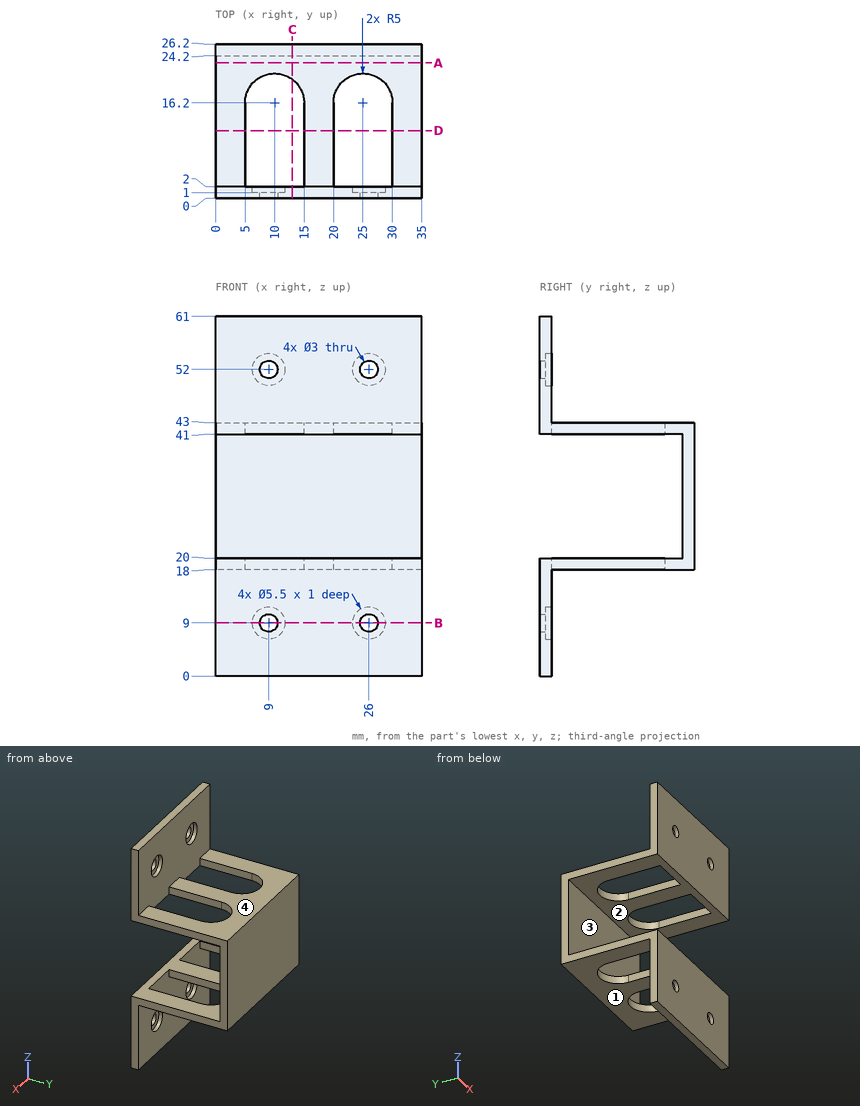
Design review of the part shown in the three views and the two pictorial views. Dimensions are in mm from the part's minimum x, y and z. Give positions to 0.01 mm unless a question says otherwise; leave off trailing zeros. Write each loop counter-clockwise with the first axis right and the second up, starting at its lowest first coordinate (ties: lowest second). Pieces come first, ordered by that corner, then holes. Notation, with made-up numbers: (7, 17) - (55, 17) arc R28 cw to (55, 47) - close; hole circle Ø9 at (44, 21). An arc over 180 degrees is marked (long way). Return JSON: item names as keys, results as strings. Group by question number.
(1) Mouldability with a two-part tool opening along Z and no side actions: class the marked faces 1, 2, 3 and 4 as +Z half, -Z half, draft (parallel to the pull), parting line (faces both ways), or undercut.
(2) We need section D-D, the plane y = 11.5. Give the boundary of the cut face in (x, z).
(3) To check wall thickness, follow probe 1 along Z at (x, y) = (26, 1.4); probe 2 along Z at (x, y) = (26, 0.6); probe 3 along X at (y, z) = (1.45, 52). State the ranges of each line that lie inside material, in increasing order.
(4) We need section A-A, the plane y = 23. Give the boundary of the cut face in (x, z), then the cut area to 3 significant figures.
(5) We need section B-B, the plane z = 9. Give the boundary of the cut face in (x, y).
(6) We need section C-C, the plane x = 13. Give the boundary of the cut face in (y, z).
(7) Insertion check: pin 1 (4.5 mm diameter, centred on x = 7.5, z = 9, fed in from +Y); pin 2 (12 mm diameter, centred on x = 15.5, y = 9.5, fed in from +Z); pin 3 (3.5 mm diameter, centred on x = 9, z = 9, fed in from +Y). Each pin has a flat end and moves straight along its axis. Give the tip position at first contact, or say it passes through.
Reported:
{
 "1": {"face 1": "-Z half", "face 2": "undercut", "face 3": "undercut", "face 4": "+Z half"},
 "2": {"outline": "(0, 18) - (5, 18) - (5, 20) - (0, 20) - close; (0, 41) - (5, 41) - (5, 43) - (0, 43) - close; (15, 18) - (20, 18) - (20, 20) - (15, 20) - close; (15, 41) - (20, 41) - (20, 43) - (15, 43) - close; (30, 18) - (35, 18) - (35, 20) - (30, 20) - close; (30, 41) - (35, 41) - (35, 43) - (30, 43) - close"},
 "3": {"probe 1": "z = 0 to 6.25, 11.75 to 20, 41 to 49.25, 54.75 to 61", "probe 2": "z = 0 to 7.5, 10.5 to 20, 41 to 50.5, 53.5 to 61", "probe 3": "x = 0 to 6.25, 11.75 to 23.25, 28.75 to 35"},
 "4": {"outline": "(0, 18) - (35, 18) - (35, 20) - (0, 20) - close; (0, 41) - (35, 41) - (35, 43) - (0, 43) - close", "area": "140 mm2"},
 "5": {"outline": "(0, 0) - (7.5, 0) - (7.5, 1) - (6.25, 1) - (6.25, 2) - (0, 2) - close; (10.5, 0) - (24.5, 0) - (24.5, 1) - (23.25, 1) - (23.25, 2) - (11.75, 2) - (11.75, 1) - (10.5, 1) - close; (27.5, 0) - (35, 0) - (35, 2) - (28.75, 2) - (28.75, 1) - (27.5, 1) - close"},
 "6": {"outline": "(0, 0) - (2, 0) - (2, 20) - (0, 20) - close; (0, 41) - (2, 41) - (2, 61) - (0, 61) - close; (20.2, 18) - (26.2, 18) - (26.2, 43) - (20.2, 43) - (20.2, 41) - (24.2, 41) - (24.2, 20) - (20.2, 20) - close"},
 "7": {"pin 1": "stops at y = 2", "pin 2": "stops at z = 43", "pin 3": "stops at y = 1"}
}
